Build history of the part. All positions in model axes, mm. A direction names the side the tool comes from. Give positions to 0.01 mm unless a question says otherwise; leave off trailing zeros. Loops run counter-clockwise (first coordinate to the right, second up) from the corner with the lowest first, then second, coordinate; pieces in that order, holes last. Notation, with made-up numbers: (-26.5, 64) - (13.5, 64) arc R9 cw to (13.5, 72) - close; hole circle Ø10 at (30.5, -22.75). An arc over 180 degrees is marked (long way). Return JSON: item names as keys, results as strings. Group by question number.
1) Mould opens along X. For faces 3 (the face through (26.5, 41, 1)), 4 (the face through (0, 20, 0)), 5 (the face through (-13.4, 27.95, 1.52)) say: released by +X, released by -X, zero draft, split by the parting line, or undercut.
2) Slice it at B-B (x = 0). List the corners of the cut face in (y, z), and give its area (3 significant figures).
3) Slice it at D-D (y = 8.5). List the corners of the cut face in (x, z).
4) 3-axis set-ups, long thin cutter, end or side, ignore diameter. For faces 1 (the face through (-9.26, 23.62, 1.48)), 2 (the face through (-26.5, 40, 1)): which of +Z, -Z, +X, -X, +Y, -Y reach the whole face in a straight line?
5) Slice it at A-A (y = 41). List the corners of the cut face in (x, z) (3 decimals), and give its area (3 significant figures).
6) Slice it at C-C (x = -7). List the corners of the cut face in (y, z) (1 decimal), and give its area (3 significant figures).
7) Drop flat-ended pins along their axis: pin 1 (1 mm diameter, centred on x = 15.5, z = 0.5, fed in from -Y); pin 2 (3 mm diameter, centred on x = -12, y = 12, fed in from +Z). Give the stop position or say it passes through.
8) Drill centre lines: probe 1 along X at (y, z) = (41, 1.05) (3 decimals); probe 2 along Y at (x, z) = (17.5, 1.4); probe 3 along Y at (x, z) = (-17, 2.5). Where is each one in solid material? Low to high. Write a range as from..to.
```python
from build123d import *

# Parameters (mm, degrees)
EXTRUDE_2_DEPTH          = 3
FILLET_3_R               = 1
SKETCH_3_R               = 13
SKETCH_3_R_2             = 1.6
CUT_EXTRUDE_5_DEPTH      = 3
CUT_EXTRUDE_6_DEPTH      = 54.17189107
CUT_EXTRUDE_6_DEPTH_BACK = 54.17189107
SKETCH_4_R               = 1.525
CUT_EXTRUDE_7_DEPTH      = 10
FILLET_4_R               = 1.5


with BuildPart() as part:
    # 草圖2 → 填料-伸長2 (new body)
    with BuildSketch(Plane.XY):
        with BuildLine():
            Line((-26.5, 46), (26.5, 46))
            Line((26.5, 46), (26.5, 36))
            Line((26.5, 36), (23, 0))
            ThreePointArc((23, 0), (0, -23), (-23, 0))
            Line((-23, 0), (-26.5, 36))
            Line((-26.5, 36), (-26.5, 46))
        make_face()
    extrude(amount=EXTRUDE_2_DEPTH)

    # 圓角3
    # the kernel refuses this fillet: 1 mm, written as the material it takes off along each edge
    with BuildSketch(Plane(origin=(-26.5, 46, -2.5), x_dir=(0, -1, 0), z_dir=(0, 0, 1)), Plane(origin=(26.5, 46, -2.5), x_dir=(-1, 0, 0), z_dir=(0, 0, 1))) as fillet_3_piece_1:
        with BuildLine():
            CenterArc((FILLET_3_R, FILLET_3_R), FILLET_3_R, 180, 90)
            Line((0, FILLET_3_R), (0, 0))
            Line((0, 0), (FILLET_3_R, 0))
        make_face()
    extrude(amount=8, mode=Mode.SUBTRACT)
    with BuildSketch(Plane(origin=(26.5, 36, -0.121241952), x_dir=(0, 1, 0), z_dir=(0, 0, 1)), Plane(origin=(-26.5, 36, -0.121241952), x_dir=(0.0967659740606196, -0.9953071617667079, 0), z_dir=(0, 0, 1))) as fillet_3_piece_2:
        with BuildLine():
            CenterArc((FILLET_3_R * 0.0484967808039, FILLET_3_R), FILLET_3_R, 264.447028967, 5.552971033)
            Line((-FILLET_3_R * 0.0482691932568, FILLET_3_R * 0.0046928382333), (0, 0))
            Line((0, 0), (FILLET_3_R * 0.0484967808039, 0))
        make_face()
    extrude(amount=3.242483904, mode=Mode.SUBTRACT)

    # 草圖3 → 除料-伸長5 (cut)
    with BuildSketch(Plane.XY):
        Circle(SKETCH_3_R)
        with Locations((18.009998301, 0)):
            Circle(SKETCH_3_R_2)
        with Locations((0, -18.009998301)):
            Circle(SKETCH_3_R_2)
        with Locations((-18.009998301, 0)):
            Circle(SKETCH_3_R_2)
        with Locations((0, 18.009998301)):
            Circle(SKETCH_3_R_2)
        with Locations((11.999602077, 11.999602077)):
            Circle(SKETCH_3_R_2)
        with Locations((11.999602077, -11.999602077)):
            Circle(SKETCH_3_R_2)
        with Locations((-11.999602077, -11.999602077)):
            Circle(SKETCH_3_R_2)
        with Locations((-11.999602077, 11.999602077)):
            Circle(SKETCH_3_R_2)
    extrude(amount=CUT_EXTRUDE_5_DEPTH, mode=Mode.SUBTRACT)

    # 草圖4 → 除料-伸長6 (cut, two sides: drawn at the far end of the back side and taken through both)
    with BuildSketch(Plane.XY.offset(-CUT_EXTRUDE_6_DEPTH_BACK)):
        with Locations((21, 41)):
            Circle(SKETCH_4_R)
        with Locations((7, 41)):
            Circle(SKETCH_4_R)
        with Locations((-7, 41)):
            Circle(SKETCH_4_R)
        with Locations((-21, 41)):
            Circle(SKETCH_4_R)
    extrude(amount=CUT_EXTRUDE_6_DEPTH + CUT_EXTRUDE_6_DEPTH_BACK, mode=Mode.SUBTRACT)

    # 草圖5 → 除料-伸長7 (cut)
    with BuildSketch(Plane.XY.offset(3)):
        Polygon((-21.5, 35), (-6.5, 35), (-20.2, 21), align=None)
        Polygon((11.3, 22.7), (-11.3, 22.7), (0, 34.95), align=None)
        Polygon((6.5, 35), (20.2, 21), (21.5, 35), align=None)
    extrude(amount=-CUT_EXTRUDE_7_DEPTH, mode=Mode.SUBTRACT)

    # 圓角4
    fillet_4_edges = [part.edges().sort_by_distance(p)[0] for p in [
        (6.5, 35, 1.5),
        (21.5, 35, 1.5),
        (20.2, 21, 1.5),
        (-11.3, 22.7, 1.5),
        (0, 34.95, 1.5),
        (11.3, 22.7, 1.5),
        (-20.2, 21, 1.5),
        (-21.5, 35, 1.5),
        (-6.5, 35, 1.5),
    ]]
    fillet(fillet_4_edges, radius=FILLET_4_R)


solid = part.part
```
Results:
{
 "1": {"face 3": "released by +X", "face 4": "zero draft", "face 5": "undercut"},
 "2": {"outline": "(-23, 0) - (-19.61, 0) - (-19.61, 3) - (-23, 3) - close; (-16.41, 0) - (-13, 0) - (-13, 3) - (-16.41, 3) - close; (13, 0) - (16.41, 0) - (16.41, 3) - (13, 3) - close; (19.61, 0) - (22.7, 0) - (22.7, 3) - (19.61, 3) - close; (34.24, 0) - (46, 0) - (46, 3) - (34.24, 3) - close", "area": "75.2 mm2"},
 "3": {"outline": "(-23.83, 0) - (-9.84, 0) - (-9.84, 3) - (-23.83, 3) - close; (9.84, 0) - (23.83, 0) - (23.83, 3) - (9.84, 3) - close"},
 "4": {"face 1": "+Z, -Z", "face 2": "+Z, -Z, -X, +Y, -Y"},
 "5": {"outline": "(-26.5, 0) - (-22.525, 0) - (-22.525, 3) - (-26.5, 3) - close; (-19.475, 0) - (-8.525, 0) - (-8.525, 3) - (-19.475, 3) - close; (-5.475, 0) - (5.475, 0) - (5.475, 3) - (-5.475, 3) - close; (8.525, 0) - (19.475, 0) - (19.475, 3) - (8.525, 3) - close; (22.525, 0) - (26.5, 0) - (26.5, 3) - (22.525, 3) - close", "area": "122 mm2"},
 "6": {"outline": "(-21.9, 0) - (-11, 0) - (-11, 3) - (-21.9, 3) - close; (11, 0) - (22.7, 0) - (22.7, 3) - (11, 3) - close; (27.4, 0) - (39.5, 0) - (39.5, 3) - (27.4, 3) - close; (42.5, 0) - (46, 0) - (46, 3) - (42.5, 3) - close", "area": "115 mm2"},
 "7": {"pin 1": "y = -17.44", "pin 2": "through"},
 "8": {"probe 1": "-26.5..-22.525, -19.475..-8.525, -5.475..5.475, 8.525..19.475, 22.525..26.5", "probe 2": "-14.92..-1.52, 1.52..23.76, 35..46", "probe 3": "-15.49..-1.24, 1.24..24.27, 35..46"}
}
